Source: CAD feature listing. Evaluate the final solid. Frame: model axes, mm. Round coordinates to 2 decimals unless told otherwise and drop trailing zeros. Loops run counter-clockwise (first coordinate to the right, second up) from the corner with the lowest first, then second, coordinate; pieces in that order, holes last.
Item 1: Section query A-A on x = 44.5. Return loops of the section in (y, z), then the cut area to 4 significant figures.
Item 2: Section query C-C on z = 82. Return loops of the section in (x, y), then the cut area to 3 significant figures.
Item 3: Ray query, L1, parallel to Z at x = 0, y = -6.25. Return the intervals inside material, ascending.
Item 4: Pull-direction query (Z, two-part tool) for faces 1 (the cylindrical face through (46.81, -12.32, 81.04)), 2 (the flat face through (-1, -12, 90)), 3 (the flat face through (-1, -12, -90)); classes: released by +Z, released by -Z, zero draft, split by the parting line, or undercut.
Item 5: Section query B-B on z = -62.5. Return loops of the section in (x, y).
Item 6: First-contact query: P1, Ø4.5, axis at x = 44.5, z = 82, coming from the -Y side; P2, Ø6.5, axis at x = 0, z = -62.5, coming from the -Y side. Flat tips, straight axial feed; report the tip coordinate or a pass-through.
```python
from build123d import *

# Parameters (mm, degrees)
F0_W     = 126
F0_H     = 180
F0_R     = 2.5
F1_DEPTH = 25


with BuildPart() as f1:
    # F0 (on Front) → F1 (new body)
    with BuildSketch(Plane.XZ):
        Rectangle(F0_W, F0_H)
        with Locations((0, -62.5)):
            Circle(F0_R, mode=Mode.SUBTRACT)
        with Locations((-44.5, 82)):
            Circle(F0_R, mode=Mode.SUBTRACT)
        with Locations((44.5, 82)):
            Circle(F0_R, mode=Mode.SUBTRACT)
    extrude(amount=F1_DEPTH)


solid = f1.part
```
Data:
1. outline: (-25, -90) - (0, -90) - (0, 79.5) - (-25, 79.5) - close; (-25, 84.5) - (0, 84.5) - (0, 90) - (-25, 90) - close
1. area: 4,375 mm2
2. outline: (-63, -25) - (-47, -25) - (-47, 0) - (-63, 0) - close; (-42, -25) - (42, -25) - (42, 0) - (-42, 0) - close; (47, -25) - (63, -25) - (63, 0) - (47, 0) - close
2. area: 2,900 mm2
3. L1: z = -90 to -65, -60 to 90
4. face 1: undercut
4. face 2: released by +Z
4. face 3: released by -Z
5. outline: (-63, -25) - (-2.5, -25) - (-2.5, 0) - (-63, 0) - close; (2.5, -25) - (63, -25) - (63, 0) - (2.5, 0) - close
6. P1: passes through
6. P2: stops at y = -25
